from build123d import *

# Parameters (mm, degrees)
CROQUIS1_R                 = 5
SALIENTE_EXTRUIR1_DEPTH    = 800
CROQUIS2_R                 = 3.5
CORTAR_EXTRUIR1_DEPTH      = 801
CROQUIS3_R                 = 6
SALIENTE_EXTRUIR2_DEPTH    = 1
CROQUIS4_R                 = 3.5
CORTAR_EXTRUIR3_DEPTH      = 1
CHAFL_N1_SIZE              = 1
CROQUIS5_W                 = 13.367882917
CROQUIS5_H                 = 1.687826657
CORTAR_EXTRUIR4_DEPTH      = 7
CORTAR_EXTRUIR4_DEPTH_BACK = 7


with BuildPart() as part:
    # Croquis1 → Saliente-Extruir1 (new body)
    with BuildSketch(Plane(origin=(0, 0, 0), x_dir=(1, 0, 0), z_dir=(0, 1, 0))):
        Circle(CROQUIS1_R)
    extrude(amount=SALIENTE_EXTRUIR1_DEPTH)

    # Croquis2 → Cortar-Extruir1 (cut, through all)
    with BuildSketch(Plane.XZ):
        Circle(CROQUIS2_R)
    extrude(amount=-CORTAR_EXTRUIR1_DEPTH, mode=Mode.SUBTRACT)

    # Croquis3 → Saliente-Extruir2 (add)
    with BuildSketch(Plane(origin=(0, 800, 0), x_dir=(1, 0, 0), z_dir=(0, 1, 0))):
        Circle(CROQUIS3_R)
    extrude(amount=SALIENTE_EXTRUIR2_DEPTH)

    # Croquis4 → Cortar-Extruir3 (cut)
    with BuildSketch(Plane(origin=(0, 801, 0), x_dir=(1, 0, 0), z_dir=(0, 1, 0))):
        Circle(CROQUIS4_R)
    extrude(amount=-CORTAR_EXTRUIR3_DEPTH, mode=Mode.SUBTRACT)

    # Chaflán1
    chafl_n1_edges = [part.edges().sort_by_distance(p)[0] for p in [
        (-3.5, 801, 0),
    ]]
    chamfer(chafl_n1_edges, length=CHAFL_N1_SIZE)

    # Croquis5 → Cortar-Extruir4 (cut, two sides)
    with BuildSketch(Plane.XY) as cortar_extruir4_sk:
        with Locations((0.334446828, 800.843913329)):
            Rectangle(CROQUIS5_W, CROQUIS5_H)
    extrude(amount=CORTAR_EXTRUIR4_DEPTH, mode=Mode.SUBTRACT)
    extrude(cortar_extruir4_sk.sketch, amount=-CORTAR_EXTRUIR4_DEPTH_BACK, mode=Mode.SUBTRACT)

    # Croquis6 → Revolución1 (revolve)
    with BuildSketch(Plane.XY):
        Polygon((-3.5, 800), (-3.5, 804.5), (-4, 805), (-5, 805), (-4.26, 804.25), (-4.26, 800), align=None)
    revolve(axis=Axis((0, 810.031166981, 0), (0, -1, 0)))


solid = part.part
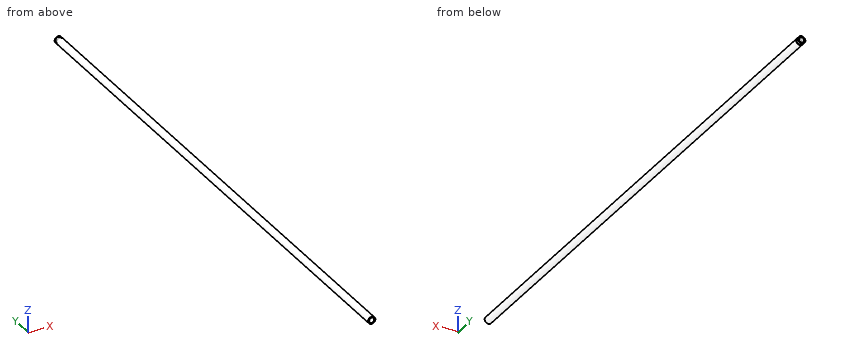
Model file for the job. Use its own axes, mm. Coordinates: 2 decimals unless noted, no trailing zeros. Order: outer loops, then holes, each group sorted by start corner. A loop starts at its lowest first (then second) coordinate and runs counter-clockwise, first axis right, second up. Notation, with made-up numbers: (43, 21) -> (58, 21) arc R18 cw to (58, 35) -> close; hole circle Ø9 at (41.25, 78.25). An arc over 180 degrees is marked (long way). Return JSON: item names as keys, results as strings. Group by question number.
Item 1: Flat gauge pins, fed straight in: P1, Ø2, axis at x = -3, y = 124.5, coming from the -Z side; P2, Ø2, axis at x = 3, y = 634.5, coming from the +Z side; P3, Ø5, axis at x = -3.5, y = 475, coming from the +Z side. Where does each tip first touch, or does it go through?
Item 2: Saw through at C-C on y = 345. Write the cut outline in (x, z), then the cut area to 3 significant figures.
Item 3: Saw through at B-B on z = 0. Write the cut outline in (x, y), then the cut area to 3 significant figures.
Item 4: Wall check: line 1 along X through (y, z) = (803.15, 0); line 2 along X through (y, z) = (144, -0.5); line 3 along Y through (x, z) = (-0.5, 4.5). Give the ranges that are in metal, low to high. Write a range as [from, to].
Item 5: Saw through at A-A on x = 0. Write the cut outline in (y, z).
Values found:
{
 "1": {"P1": "stops at z = -4.58", "P2": "stops at z = 4.58", "P3": "stops at z = 4.9"},
 "2": {"outline": "circle Ø10 at (0, 0); hole circle Ø7 at (0, 0)", "area": "40.1 mm2"},
 "3": {"outline": "(-5, 0) -> (-3.5, 0) -> (-3.5, 804.5) -> (-4, 805) -> (-5, 805) -> (-4.26, 804.25) -> (-4.26, 800) -> (-5, 800) -> close; (3.5, 0) -> (5, 0) -> (5, 800) -> (4.26, 800) -> (4.26, 804.25) -> (5, 805) -> (4, 805) -> (3.5, 804.5) -> close", "area": "2,410 mm2"},
 "4": {"line 1": "x = [-4.26, -3.5], [3.5, 4.26]", "line 2": "x = [-4.97, -3.46], [3.46, 4.97]", "line 3": "y = [0, 800], [804.52, 805]"},
 "5": {"outline": "(0, -5) -> (800, -5) -> (800, -4.26) -> (804.25, -4.26) -> (805, -5) -> (805, -4) -> (804.5, -3.5) -> (0, -3.5) -> close; (0, 3.5) -> (804.5, 3.5) -> (805, 4) -> (805, 5) -> (804.25, 4.26) -> (800, 4.26) -> (800, 5) -> (0, 5) -> close"}
}
